Geometry check sheet. Reference: drawing and pictorial views, mm from the part's lowest x, y, z. A direction names the side the tool comes from. Round coordinates to 2 decimals unless told otherwise and drop trailing zeros. Loops run counter-clockwise (first coordinate to the right, second up) from the corner with the lowest first, then second, coordinate; pieces in that order, holes last. Notation, with made-up numbers: (13, -23) -> (60, -23) arc R15 cw to (60, -13) -> close; hole circle Ø9 at (33, 39.25). An arc over 180 degrees is marked (long way). Write item = value, one per line.
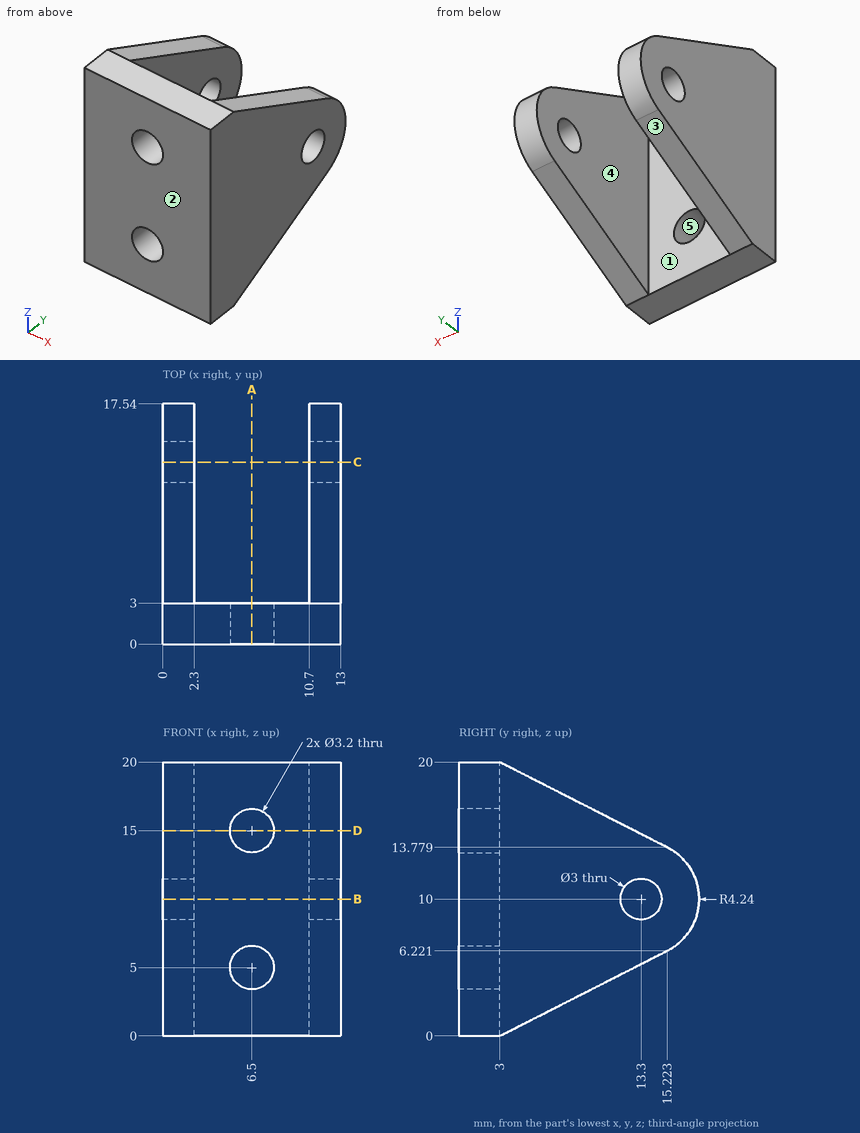
(1) Go/stop test with flat-tipped pins: pin 1 Ø2 at (x, z) = (8, 5) entering from +Y; pin 2 Ø3 at (x, z) = (3, 3) entering from +Y; pin 3 Ø4 at (x, y) = (8.5, 11.5) entering from -Z; pin 4 Ø2 at (x, z) = (10.5, 3) entering from +Y. Record where each tip stops, or that it passes through.
Filled sheet:
pin_1 = 3
pin_2 = 11.5
pin_3 = through
pin_4 = 10.82
(2) Draft check along Z on the marked faces 3, 4 and 5. Enter one of: released by +Z, released by -Z, zero draft, split by the parting line, or undercut.
Filled sheet:
face_3 = released by -Z
face_4 = zero draft
face_5 = undercut
(3) Sectioned sample at B-B, the plane z = 10. Record the cut outline in (x, y).
Filled sheet:
outline = (0, 0) -> (13, 0) -> (13, 11.8) -> (10.7, 11.8) -> (10.7, 3) -> (2.3, 3) -> (2.3, 11.8) -> (0, 11.8) -> close; (0, 14.8) -> (2.3, 14.8) -> (2.3, 17.54) -> (0, 17.54) -> close; (10.7, 14.8) -> (13, 14.8) -> (13, 17.54) -> (10.7, 17.54) -> close
(4) Sectioned sample at C-C, the plane y = 13.3. Record the cut outline in (x, z).
Filled sheet:
outline = (0, 5.24) -> (2.3, 5.24) -> (2.3, 8.5) -> (0, 8.5) -> close; (0, 11.5) -> (2.3, 11.5) -> (2.3, 14.76) -> (0, 14.76) -> close; (10.7, 5.24) -> (13, 5.24) -> (13, 8.5) -> (10.7, 8.5) -> close; (10.7, 11.5) -> (13, 11.5) -> (13, 14.76) -> (10.7, 14.76) -> close
(5) Sectioned sample at D-D, the plane z = 15. Record the cut outline in (x, y).
Filled sheet:
outline = (0, 0) -> (4.9, 0) -> (4.9, 3) -> (2.3, 3) -> (2.3, 12.82) -> (0, 12.82) -> close; (8.1, 0) -> (13, 0) -> (13, 12.82) -> (10.7, 12.82) -> (10.7, 3) -> (8.1, 3) -> close
(6) Set-up check for the marked faces 1 and 2: record each of +Z, -Z, +X, -X, +Y, -Y from which the full face is reachable in a straight line by a thin tool's end or side.
Filled sheet:
face_1 = +Z, -Z, +Y
face_2 = +Z, -Z, +X, -X, -Y
(7) Sectioned sample at A-A, the plane x = 6.5. Record the cut outline in (y, z), and give its area (3 significant figures).
Filled sheet:
outline = (0, 0) -> (3, 0) -> (3, 3.4) -> (0, 3.4) -> close; (0, 6.6) -> (3, 6.6) -> (3, 13.4) -> (0, 13.4) -> close; (0, 16.6) -> (3, 16.6) -> (3, 20) -> (0, 20) -> close
area = 40.8 mm2
(8) Material ranges on probe 1 along X at (y, z) = (11, 15); probe 2 along Y at (x, z) = (4.25, 12.75); probe 3 along Y at (x, z) = (0.7, 10), recorded low to high. Write a range as from..to.
Filled sheet:
probe_1 = 0..2.3, 10.7..13
probe_2 = 0..3
probe_3 = 0..11.8, 14.8..17.54
